from build123d import *

# Parameters (mm, degrees)
SKETCH1_W                = 161
SKETCH1_H                = 100
BOSS_EXTRUDE1_DEPTH      = 12.75
BOSS_EXTRUDE1_DEPTH_BACK = 12.75
SKETCH2_R                = 6.63
SKETCH2_R_2              = 3.525
SKETCH2_R_3              = 1.975
CUT_EXTRUDE1_DEPTH       = 101
FILLET1_R                = 1
FILLET2_R                = 1
FILLET3_R                = 1
FILLET4_R                = 1
SKETCH3_R                = 2.5
BOSS_EXTRUDE2_DEPTH      = 10
SKETCH4_R                = 1.45
CUT_EXTRUDE2_DEPTH       = 5
SKETCH5_W                = 6
SKETCH5_H                = 13
CUT_EXTRUDE3_DEPTH       = 19.25
SKETCH6_R                = 10.25
CUT_EXTRUDE4_DEPTH       = 43.477415469
SKETCH8_R                = 1.5
CUT_EXTRUDE5_DEPTH       = 36.5
SKETCH11_R               = 3
BOSS_EXTRUDE4_DEPTH      = 5
SKETCH12_R               = 1.5
CUT_EXTRUDE7_DEPTH       = 5
SKETCH13_W               = 18.75
SKETCH13_H               = 6
BOSS_EXTRUDE5_DEPTH      = 100
SKETCH14_W               = 4
SKETCH14_H               = 2
BOSS_EXTRUDE6_DEPTH      = 25
BOSS_EXTRUDE6_DEPTH_BACK = 125


with BuildPart() as part:
    # Sketch1 → Boss-Extrude1 (new body, two sides)
    with BuildSketch(Plane(origin=(0, 0, 0), x_dir=(1, 0, 0), z_dir=(0, 1, 0))) as boss_extrude1_sk:
        Rectangle(SKETCH1_W, SKETCH1_H)
    extrude(amount=BOSS_EXTRUDE1_DEPTH)
    extrude(boss_extrude1_sk.sketch, amount=-BOSS_EXTRUDE1_DEPTH_BACK)

    # Sketch2 → Cut-Extrude1 (cut, through all)
    with BuildSketch(Plane.XY.offset(50)):
        with Locations((-67.75, 0)):
            Circle(SKETCH2_R)
        with Locations((67.75, 0)):
            Circle(SKETCH2_R_2)
        with Locations((-75.45, 8.2)):
            Circle(SKETCH2_R_3)
        with Locations((-75.45, -8.2)):
            Circle(SKETCH2_R_3)
        with Locations((-60.05, -8.2)):
            Circle(SKETCH2_R_3)
        with Locations((-60.05, 8.2)):
            Circle(SKETCH2_R_3)
    extrude(amount=-CUT_EXTRUDE1_DEPTH, mode=Mode.SUBTRACT)

    # Fillet1
    fillet1_edges = [part.edges().sort_by_distance(p)[0] for p in [
        (-74.38, 0, -50),
    ]]
    fillet(fillet1_edges, radius=FILLET1_R)

    # Fillet2
    fillet2_edges = [part.edges().sort_by_distance(p)[0] for p in [
        (-74.38, 0, 50),
    ]]
    fillet(fillet2_edges, radius=FILLET2_R)

    # Fillet3
    fillet3_edges = [part.edges().sort_by_distance(p)[0] for p in [
        (64.225, 0, 50),
    ]]
    fillet(fillet3_edges, radius=FILLET3_R)

    # Fillet4
    fillet4_edges = [part.edges().sort_by_distance(p)[0] for p in [
        (64.225, 0, -50),
    ]]
    fillet(fillet4_edges, radius=FILLET4_R)

    # Sketch3 → Boss-Extrude2 (add)
    with BuildSketch(Plane(origin=(0, 12.75, 0), x_dir=(1, 0, 0), z_dir=(0, 1, 0))):
        with Locations((-16.76, 42.46)):
            Circle(SKETCH3_R)
        with Locations((58.37, 42.46)):
            Circle(SKETCH3_R)
        with Locations((-17, -5.8)):
            Circle(SKETCH3_R)
        with Locations((34.7, -0.9)):
            Circle(SKETCH3_R)
        with Locations((65.72, -5.8)):
            Circle(SKETCH3_R)
    extrude(amount=BOSS_EXTRUDE2_DEPTH)

    # Sketch4 → Cut-Extrude2 (cut)
    with BuildSketch(Plane(origin=(0, 22.75, 0), x_dir=(1, 0, 0), z_dir=(0, 1, 0))):
        with Locations((-16.76, 42.46)):
            Circle(SKETCH4_R)
        with Locations((-17, -5.8)):
            Circle(SKETCH4_R)
        with Locations((34.7, -0.9)):
            Circle(SKETCH4_R)
        with Locations((65.72, -5.8)):
            Circle(SKETCH4_R)
        with Locations((58.37, 42.46)):
            Circle(SKETCH4_R)
    extrude(amount=-CUT_EXTRUDE2_DEPTH, mode=Mode.SUBTRACT)

    # Sketch5 → Cut-Extrude3 (cut)
    with BuildSketch(Plane(origin=(80.5, 0, 0), x_dir=(0, 0, -1), z_dir=(1, 0, 0))):
        with Locations((-30, 0)):
            Rectangle(SKETCH5_W, SKETCH5_H)
        with Locations((-10, 0)):
            Rectangle(SKETCH5_W, SKETCH5_H)
        with Locations((10, 0)):
            Rectangle(SKETCH5_W, SKETCH5_H)
        with Locations((30, 0)):
            Rectangle(SKETCH5_W, SKETCH5_H)
    extrude(amount=-CUT_EXTRUDE3_DEPTH, mode=Mode.SUBTRACT)

    # Sketch6 → Cut-Extrude4 (cut, through all)
    with BuildSketch(Plane(origin=(0, 20.916044041, 3.688062894), x_dir=(1, 0, 0), z_dir=(0, 0.984807753, 0.173648178))):
        with Locations((0, -21.249093385)):
            Circle(SKETCH6_R)
    extrude(amount=-CUT_EXTRUDE4_DEPTH, mode=Mode.SUBTRACT)

    # Sketch8 → Cut-Extrude5 (cut, through all)
    with BuildSketch(Plane.XZ.offset(12.75)):
        with Locations((28.5, 2.93086019)):
            Circle(SKETCH8_R)
        with Locations((28.5, 45.38111272)):
            Circle(SKETCH8_R)
        with Locations((-28.5, 2.93086019)):
            Circle(SKETCH8_R)
        with Locations((-28.5, 45.38111272)):
            Circle(SKETCH8_R)
    extrude(amount=-CUT_EXTRUDE5_DEPTH, mode=Mode.SUBTRACT)

    # Sketch11 → Boss-Extrude4 (add)
    with BuildSketch(Plane(origin=(0, 12.75, 0), x_dir=(1, 0, 0), z_dir=(0, 1, 0))):
        with Locations((-38, -6.5)):
            Circle(SKETCH11_R)
        with Locations((-38, -44)):
            Circle(SKETCH11_R)
        with Locations((-75.5, -6.5)):
            Circle(SKETCH11_R)
        with Locations((-75.5, -44)):
            Circle(SKETCH11_R)
    extrude(amount=BOSS_EXTRUDE4_DEPTH)

    # Sketch12 → Cut-Extrude7 (cut)
    with BuildSketch(Plane(origin=(0, 17.75, 0), x_dir=(1, 0, 0), z_dir=(0, 1, 0))):
        with Locations((-75.5, -44)):
            Circle(SKETCH12_R)
        with Locations((-75.5, -6.5)):
            Circle(SKETCH12_R)
        with Locations((-38, -6.5)):
            Circle(SKETCH12_R)
        with Locations((-38, -44)):
            Circle(SKETCH12_R)
    extrude(amount=-CUT_EXTRUDE7_DEPTH, mode=Mode.SUBTRACT)

    # Sketch13 → Boss-Extrude5 (add)
    with BuildSketch(Plane.XY.offset(50)):
        with Locations((89.875, 9.75)):
            Rectangle(SKETCH13_W, SKETCH13_H)
    extrude(amount=-BOSS_EXTRUDE5_DEPTH)

    # Sketch14 → Boss-Extrude6 (add, two sides)
    with BuildSketch(Plane.XY.offset(50)) as boss_extrude6_sk:
        with Locations((101.25, 11.75)):
            Rectangle(SKETCH14_W, SKETCH14_H)
    extrude(amount=BOSS_EXTRUDE6_DEPTH)
    extrude(boss_extrude6_sk.sketch, amount=-BOSS_EXTRUDE6_DEPTH_BACK)


solid = part.part
Design review of the part built by this model. Coordinates are the model's own, in mm. A direction names the side the tool comes from. Round coordinates to 2 decimals unless told otherwise and drop trailing zeros. Loops run counter-clockwise (first coordinate to the right, second up) from the corner with the lowest first, then second, coordinate; pieces in that order, holes last. Notation, with made-up numbers: (69, -23) - (94, -23) arc R16 cw to (94, -13) - close; hole circle Ø2 at (69.5, -36). An arc over 180 degrees is marked (long way). One line per question, with ' | ' between items.
1. Draft analysis for pull direction Y (two halves, no side actions). For faces 5 (the face through (90, 6.75, 1)), 6 (the face through (-73.011, -4.034, 0.686)), 7 (the face through (80.5, -3, 1)), state which applies: released by +Y, released by -Y, zero draft, split by the parting line, or undercut.
Results are:
face 5: released by -Y | face 6: undercut | face 7: zero draft
2. For faces 1 (the face through (71.1, 1.1, 20.1)), 2 (the face through (73, 0, 7)), 3 (the face through (101, 10.75, 1)), 4 (the face through (8, 0, 50)), list the 3-axis set-ups (+Z, -Z, +X, -X, +Y, -Y) from which the entire face can be reached by the end or side of a thin tool; tool diameter is ignored.
Results are:
face 1: +Z, -Z | face 2: +X | face 3: +Z, -Z, +X, -Y | face 4: +Z, -X, +Y, -Y
3. For L1, parallel to X at y = 15, z = 44; L2, parallel to Y at x = -60, z = 16; L3, parallel to X at y = -1, z = 36.5, list the stretches that pass through material, from the lowest coordinate up. Write a range as [from, to].
Results are:
L1: x = [-78.5, -77], [-74, -72.5], [-41, -39.5], [-36.5, -35] | L2: y = [-12.75, -10.17], [-6.23, 6.23], [10.17, 12.75] | L3: x = [-80.5, -74.3], [-61.2, 64.37], [71.13, 80.5]
4. We need section B-B, the plane z = -29. State the section outline as (x, y) points (3 decimals), and give its area (3 significant figures).
Results are:
outline: (-80.5, -12.75) - (80.5, -12.75) - (80.5, -6.5) - (61.25, -6.5) - (61.25, 6.5) - (80.5, 6.5) - (80.5, 6.75) - (99.25, 6.75) - (99.25, 10.75) - (103.25, 10.75) - (103.25, 12.75) - (-80.5, 12.75) - close; hole circle Ø3.95 at (-75.45, -8.2); hole circle Ø3.95 at (-75.45, 8.2); hole circle Ø13.26 at (-67.75, 0); hole circle Ø3.95 at (-60.05, -8.2); hole circle Ø3.95 at (-60.05, 8.2) | area: 3,790 mm²
5. Clearance check with flat-ended pins moving along their axes: P1, Ø1.8, axis at x = -76, z = 43.5, coming from the +Y side; P2, Ø10, axis at y = -3.5, z = 53.5, coming from the +X side; P3, Ø3, axis at x = -75.45, y = 8.2, coming from the -Z side; P4, Ø3, axis at y = -0.5, z = -30.5, coming from the +X side. State where each tip first meets the part, or that it passes through.
Results are:
P1: stops at y = 17.75 | P2: stops at x = 80.5 | P3: passes through | P4: stops at x = 61.25
6. We need section C-C, the plane x = 75. State the section outline as (y, z) points.
Results are:
outline: (-12.75, -50) - (12.75, -50) - (12.75, 50) - (-12.75, 50) - close; hole (-6.5, -33) - (6.5, -33) - (6.5, -27) - (-6.5, -27) - close; hole (-6.5, -13) - (6.5, -13) - (6.5, -7) - (-6.5, -7) - close; hole (-6.5, 7) - (6.5, 7) - (6.5, 13) - (-6.5, 13) - close; hole (-6.5, 27) - (6.5, 27) - (6.5, 33) - (-6.5, 33) - close
7. We need section A-A, the plane x = -67.75. State the section outline as (y, z) points, and give its area (3 significant figures).
Results are:
outline: (-12.75, -50) - (-7.63, -50) arc R1 ccw to (-6.63, -49) - (-6.63, 49) arc R1 ccw to (-7.63, 50) - (-12.75, 50) - close; (6.63, -49) arc R1 ccw to (7.63, -50) - (12.75, -50) - (12.75, 50) - (7.63, 50) arc R1 ccw to (6.63, 49) - close | area: 1,220 mm²
8. We need section D-D, the plane x = -7. State the section outline as (y, z) points.
Results are:
outline: (-12.75, -50) - (12.75, -50) - (12.75, 16.22) - (-12.75, 11.73) - close; (-12.75, 26.93) - (12.75, 31.43) - (12.75, 50) - (-12.75, 50) - close
